Build history of the part. All positions in model axes, mm. Face numbers are marked on the shaded views. A direction names the side the tool comes from. Give positions to 0.01 mm unless a question says otherwise; leave off trailing zeros. Loops run counter-clockwise (first coordinate to the right, second up) from the corner with the lowest first, then second, coordinate; pieces in that order, holes last. Notation, with made-up numbers: (-9.5, 15) -> (12.5, 15) arc R19 ccw to (12.5, 20) -> close; hole circle Ø10 at (58.25, -27). An arc over 180 degrees is marked (long way). Answer in a Markdown table with one row per item. Add a question column.
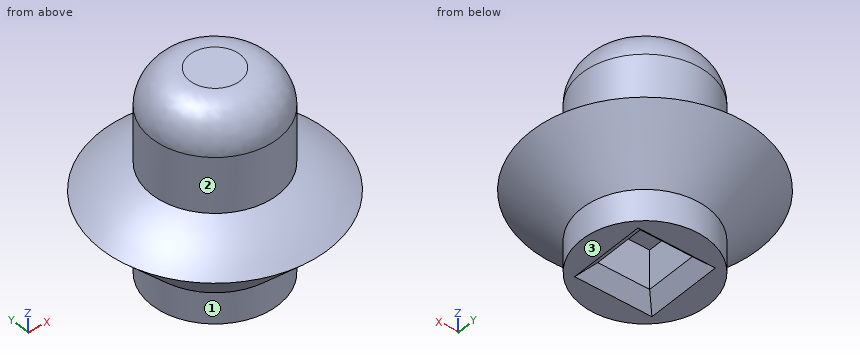
from build123d import *

# Parameters (mm, degrees)
SKETCH036_W     = 2.05
SKETCH036_H     = 2.05
POCKET015_DEPTH = 5
CHAMFER006_SIZE = 0.5


with BuildPart() as part:
    # Sketch035 (on DatumPlane) → Revolution (revolve)
    with BuildSketch(Plane(origin=(100, 13, 0), x_dir=(1, 0, 0), z_dir=(0, -1, 0))):
        with BuildLine():
            ThreePointArc((-2.5, 7.3), (-3.544517, 6.819494), (-4.5, 6.18))
            Line((-4.5, 6.18), (-2.5, 4.18))
            Line((-2.5, 4.18), (-2.5, 2.95))
            Line((-2.5, 2.95), (0, 2.95))
            Line((0, 11), (0, 2.95))
            Line((-1, 11), (0, 11))
            ThreePointArc((-1, 11), (-2.06066, 10.56066), (-2.5, 9.5))
            Line((-2.5, 7.3), (-2.5, 9.5))
        make_face()
    revolve(axis=Axis((100, 13, 0), (0, 0, 1)))

    # Sketch036 → Pocket015 (cut)
    with BuildSketch(Plane.XY):
        with Locations((100, 13)):
            Rectangle(SKETCH036_W, SKETCH036_H)
    extrude(amount=POCKET015_DEPTH, mode=Mode.SUBTRACT)

    # Chamfer006
    chamfer006_edges = [part.edges().sort_by_distance(p)[0] for p in [
        (101.025, 13, 2.95),
        (100, 14.025, 2.95),
        (98.975, 13, 2.95),
        (100, 11.975, 2.95),
    ]]
    chamfer(chamfer006_edges, length=CHAMFER006_SIZE)


solid = part.part
(1) Saw through at C-C, the plane z = 5.25. List the corners of the cut face in (x, y).
(2) 3-axis set-ups, long thin cutter, end or side, ignore diameter. For the marked faces 1, 2 and 3: which of +Z, -Z, +X, -X, +Y, -Y reach the whole face in a straight line?
(3) Wall check: line 1 along Y through (x, z) = (100, 9.5); line 2 along X through (y, z) = (13.25, 4.75) (3 decimals); line 3 along X through (y, z) = (14.5, 9.75). Give the ranges that are in metal, low to high. Write a range as from..to.
(4) Saw through at B-B, the plane z = 8.5. List the corners of the cut face in (x, y), then the cut area to 3 significant figures.
(5) Saw through at A-A, the plane z = 4. List the corners of the cut face in (x, y) (3 decimals).
(6) Flat gauge pins, fed straight in: pin 1 Ø0.5 at (x, z) = (100, 4.5) entering from +Y; pin 2 Ø2 at (x, y) = (102, 10.5) entering from +Z; pin 3 Ø3 at (x, z) = (99.5, 8) entering from +Y. Where does each tip first touch, or does it go through?
Worked answers:
| question | item | result |
|---|---|---|
| 1 | outline | circle Ø7.14 at (100, 13) |
| 2 | face 1 | -Z |
| 2 | face 2 | +Z |
| 2 | face 3 | -Z, +X, -X, +Y, -Y |
| 3 | line 1 | 10.5..15.5 |
| 3 | line 2 | 96.94..98.975, 101.025..103.06 |
| 3 | line 3 | 98.03..101.97 |
| 4 | outline | circle Ø5 at (100, 13) |
| 4 | area | 19.6 mm^2 |
| 5 | outline | circle Ø5 at (100, 13); hole (98.975, 11.975) -> (101.025, 11.975) -> (101.025, 14.025) -> (98.975, 14.025) -> close |
| 6 | pin 1 | y = 16.07 |
| 6 | pin 2 | z = 10.4 |
| 6 | pin 3 | y = 17.04 |
